Check sheet for the modelled part. Datum: model origin and axes. Units: mm. Face numbers are marked on the shaded views. A direction names the side the tool comes from. Give positions to 0.01 mm unless a question says otherwise; leave off trailing zeros. Loops run counter-clockwise (first coordinate to the right, second up) from the corner with the lowest first, then second, coordinate; pieces in that order, holes last. Notation, with made-up numbers: M 32.5,4 L 60.5,4 A24 ccw 60.5,39 Z; hole C -37,34 d4. An arc over 180 degrees is marked long. Write each question's results on one line, items separated by ' | '. Start each with the question number.
1. Material ranges on line 1 along Y through (x, z) = (-15, 5.5); line 2 along Y through (x, z) = (35, 6.75); line 3 along X through (y, z) = (10.5, 1.25), recorded low to high.
2. Draft check along X on the marked faces 1, 2 and 3. Enter one of: pulls with the +X half, pulls with the -X half, needs draft (parallel to the pull), parting line crosses it, or undercut.
3. Sectioned sample at B-B on z = 2. Give the number of separate pieces and of enclosed holes in the cut face, and give its area (3 significant figures).
4. Sectioned sample at D-D on y = 47. Record the cut outline in (x, z), and give its area (3 significant figures).
5. Go/stop test with flat-tipped pins: pin 1 (3 mm diameter, centred on y = 50, z = 8, fed in from +X); pin 2 (3.5 mm diameter, centred on y = 10.5, z = 4.5, fed in from +X); pin 3 (2 mm diameter, centred on y = 17, z = 10.5, fed in from -X). Record where each tip stops, or that it passes through.
6. Tool access check on the marked faces 4, 5, 6, 7 and 8. Record the directions out of +Z, -Z, +X, -X, +Y, -Y that give a thin tool (end or side, any length) a straight path to the whole face; none if there is none.
7. Sectioned sample at A-A on x = -15. Record the cut outline in (y, z), and give its area (3 significant figures).
8. Sectioned sample at C-C on y = 35. Record the cut outline in (x, z), and give its area (3 significant figures).
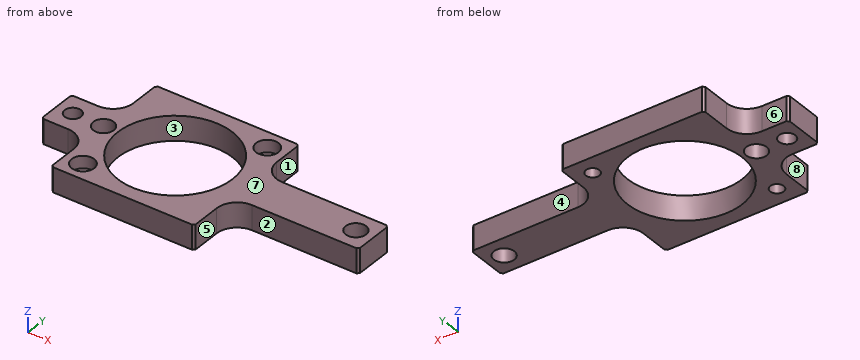
```python
from build123d import *

# Parameters (mm, degrees)
ESQUISSE4_R             = 28
BASE_EXTRUSION_DEPTH    = 12
CHANFREIN2_SIZE         = 1
PER_AGE1_D              = 6.6
PER_AGE1_CBORE_D        = 11
PER_AGE1_CBORE_DEPTH    = 6
ESQUISSE7_R             = 5
ESQUISSE7_R_2           = 4
ENL_V_MAT_EXTRU_1_DEPTH = 150.89329538


with BuildPart() as part:
    # Esquisse4 → Base-Extrusion (new body)
    with BuildSketch(Plane.XY):
        with BuildLine():
            Line((0, 0), (70, 0))
            Line((70, 0), (70, 15))
            ThreePointArc((70, 15), (72.928932188, 22.071067812), (80, 25))
            Line((80, 25), (132, 25))
            Line((132, 25), (132, 45))
            Line((132, 45), (80, 45))
            ThreePointArc((80, 45), (72.928932188, 47.928932188), (70, 55))
            Line((70, 55), (70, 70))
            Line((70, 70), (0, 70))
            Line((0, 70), (0, 55))
            ThreePointArc((0, 55), (-2.928932188, 47.928932188), (-10, 45))
            Line((-10, 45), (-23, 45))
            Line((-23, 45), (-23, 25))
            Line((-23, 25), (-10, 25))
            ThreePointArc((-10, 25), (-2.928932188, 22.071067812), (0, 15))
            Line((0, 15), (0, 0))
        make_face()
        with Locations((35, 35)):
            Circle(ESQUISSE4_R, mode=Mode.SUBTRACT)
    extrude(amount=BASE_EXTRUSION_DEPTH)

    # Chanfrein2
    chanfrein2_edges = [part.edges().sort_by_distance(p)[0] for p in [
        (-23, 45, 6),
        (-23, 25, 6),
        (0, 0, 6),
        (70, 0, 6),
        (132, 25, 6),
        (132, 45, 6),
        (70, 70, 6),
        (0, 70, 6),
    ]]
    chamfer(chanfrein2_edges, length=CHANFREIN2_SIZE)

    # Perçage1 (through all)
    with Locations(Plane.XY.offset(12)):
        with Locations((9, 9), (61, 61)):
            CounterBoreHole(PER_AGE1_D / 2, PER_AGE1_CBORE_D / 2, PER_AGE1_CBORE_DEPTH)

    # Esquisse7 → Enlèv. mat.-Extru.1 (cut, through all)
    with BuildSketch(Plane.XY.offset(12)):
        with Locations((0, 35)):
            Circle(ESQUISSE7_R)
        with Locations((-15, 35)):
            Circle(ESQUISSE7_R_2)
        with Locations((123.39, 35)):
            Circle(ESQUISSE7_R)
    extrude(amount=-ENL_V_MAT_EXTRU_1_DEPTH, mode=Mode.SUBTRACT)


solid = part.part
```
Output values:
1) line 1: 25 to 31, 39 to 45 | line 2: 0 to 7, 63 to 70 | line 3: 0 to 6.06, 11.94 to 21.44, 48.56 to 70
2) face 1: pulls with the +X half | face 2: needs draft | face 3: undercut
3) separate pieces: 1 | enclosed holes: 6 | area: 3,940 mm2
4) outline: M -4,0 L 9.7,0 L 9.7,12 L -4,12 Z; M 60.3,0 L 74,0 L 74,12 L 60.3,12 Z | area: 329 mm2
5) pin 1: x = 72.4 | pin 2: x = 70 | pin 3: x = -0.46
6) face 4: +Z, -Z, +X, +Y | face 5: +Z, -Z, +X, -Y | face 6: +Z, -Z, -X, +Y | face 7: +Z, +X, -X, +Y, -Y | face 8: +Z, -Z, -X, -Y
7) outline: M 25,0 L 31,0 L 31,12 L 25,12 Z; M 39,0 L 45,0 L 45,12 L 39,12 Z | area: 144 mm2
8) outline: M -23,0 L -19,0 L -19,12 L -23,12 Z; M -11,0 L -5,0 L -5,12 L -11,12 Z; M 5,0 L 7,0 L 7,12 L 5,12 Z; M 63,0 L 118.39,0 L 118.39,12 L 63,12 Z; M 128.39,0 L 132,0 L 132,12 L 128.39,12 Z | area: 852 mm2
